The drawing under review shows one solid part. Ordinate dimensions are in mm from its lowest x, y, z. Coordinates: 2 decimals unless noted, no trailing zeros. Loops run counter-clockwise (first coordinate to the right, second up) from the corner with the lowest first, then second, coordinate; pieces in that order, holes last. Notation, with made-up numbers: M 75,-21.75 L 105,-21.75 A21 cw 105,-4.75 Z; hole C 74.5,5.5 d6. An arc over 180 degrees is marked long. Put each result on its own line as item: value.
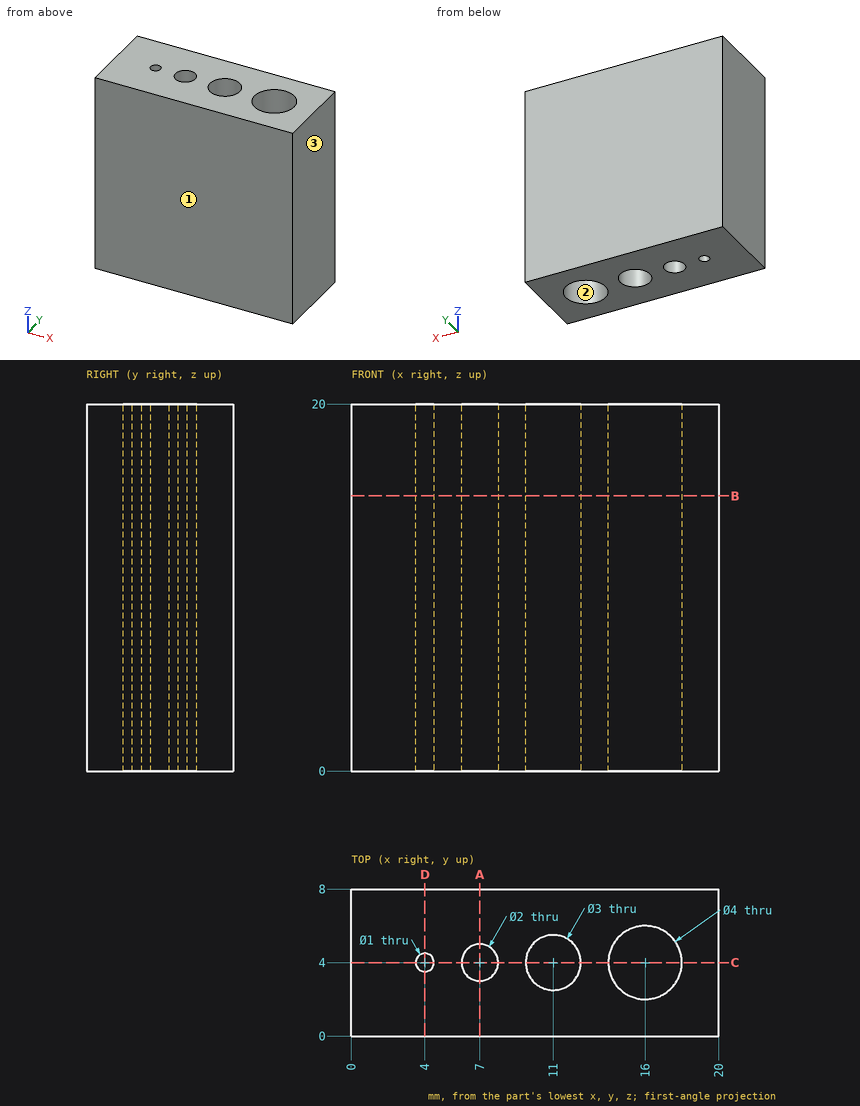
(1) Draft analysis for pull direction Y (two halves, no side actions). For the marked faces 1, 2 and 3, state which applies: +Y half, -Y half, draft (parallel to the pull), parting line (faces both ways), or undercut.
Determined:
face 1: -Y half
face 2: undercut
face 3: draft
(2) Wall thickness on line 1 along Y through (x, z) = (4, 6.75); line 2 along X through (y, z) = (3.25, 10); line 3 along Y through (x, z) = (16, 16.25): over which ranges is each line inside the solid? List them lowest first. Write a range as [from, to].
Determined:
line 1: y = [0, 3.5], [4.5, 8]
line 2: x = [0, 6.34], [7.66, 9.7], [12.3, 14.15], [17.85, 20]
line 3: y = [0, 2], [6, 8]
(3) Add section B-B (z = 15). Write out the cut boundary in (x, y).
Determined:
outline: M 0,0 L 20,0 L 20,8 L 0,8 Z; hole C 4,4 d1; hole C 7,4 d2; hole C 11,4 d3; hole C 16,4 d4
(4) For pin 1 (2.5 mm diameter, centred on x = 11, y = 4, fed in from -Z); pin 2 (2 mm diameter, centred on y = 3.5, z = 4.5, fed in from -X), all flat-tipped, find the tip position at first contact; note any pin that passes through.
Determined:
pin 1: passes through
pin 2: stops at x = 0
(5) Add section D-D (x = 4). Write out the cut boundary in (y, z).
Determined:
outline: M 0,0 L 3.5,0 L 3.5,20 L 0,20 Z; M 4.5,0 L 8,0 L 8,20 L 4.5,20 Z
(6) Add section C-C (y = 4). Write out the cut boundary in (x, z).
Determined:
outline: M 0,0 L 3.5,0 L 3.5,20 L 0,20 Z; M 4.5,0 L 6,0 L 6,20 L 4.5,20 Z; M 8,0 L 9.5,0 L 9.5,20 L 8,20 Z; M 12.5,0 L 14,0 L 14,20 L 12.5,20 Z; M 18,0 L 20,0 L 20,20 L 18,20 Z
(7) Add section A-A (x = 7). Write out the cut boundary in (y, z), plus the area to 3 significant figures.
Determined:
outline: M 0,0 L 3,0 L 3,20 L 0,20 Z; M 5,0 L 8,0 L 8,20 L 5,20 Z
area: 120 mm^2
